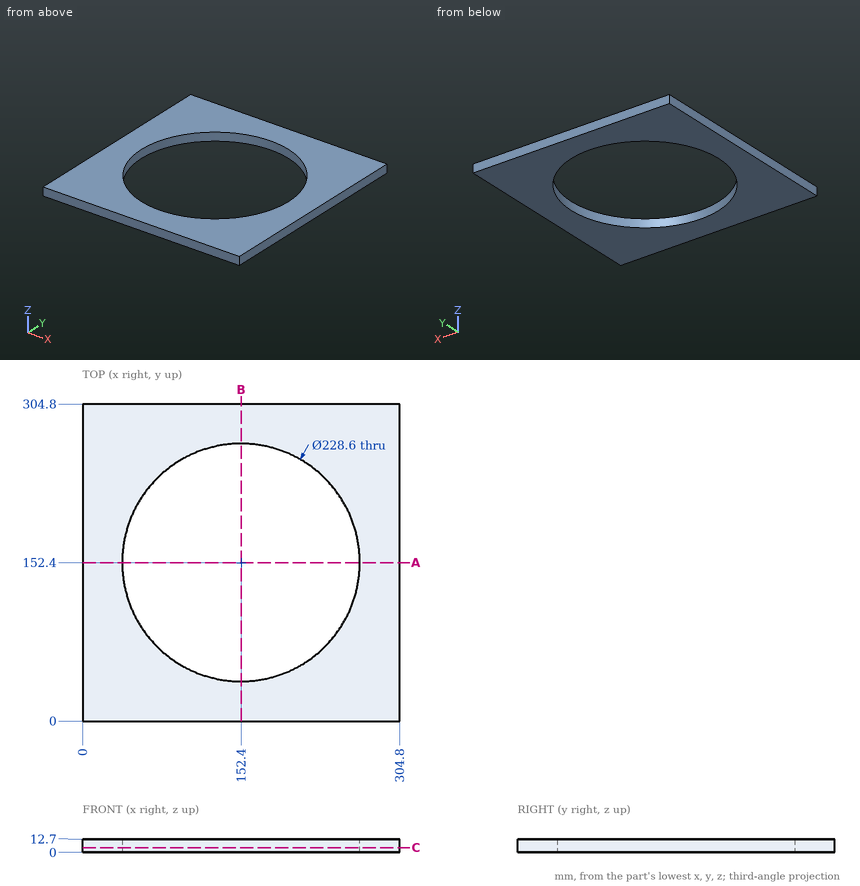
The drawing under review shows one solid part. Ordinate dimensions are in mm from its lowest x, y, z. Give positions to 0.01 mm unless a question says otherwise; leave off trailing zeros. Write each loop counter-clockwise with the first axis right and the second up, starting at its lowest first coordinate (ties: lowest second). Pieces come first, ordered by that corner, then holes.
1. Add section A-A, the plane y = 152.4. Write out the cut boundary in (x, z), plus the area to 3 significant figures.
2. Wall thickness on L1, parallel to Y at x = 152.4, z = 9.5; L2, parallel to X at y = 170.5, z = 9.75; L3, parallel to Y at x = 204.5, z = 4.25: over which ranges is each line inside the solid? List them lowest first.
3. Add section C-C, the plane z = 4.5. Write out the cut boundary in (x, y).
Worked answers:
1. outline: (0, 0) - (38.1, 0) - (38.1, 12.7) - (0, 12.7) - close; (266.7, 0) - (304.8, 0) - (304.8, 12.7) - (266.7, 12.7) - close
1. area: 968 mm2
2. L1: y = 0 to 38.1, 266.7 to 304.8
2. L2: x = 0 to 39.54, 265.26 to 304.8
2. L3: y = 0 to 50.66, 254.14 to 304.8
3. outline: (0, 0) - (304.8, 0) - (304.8, 304.8) - (0, 304.8) - close; hole circle Ø228.6 at (152.4, 152.4)
